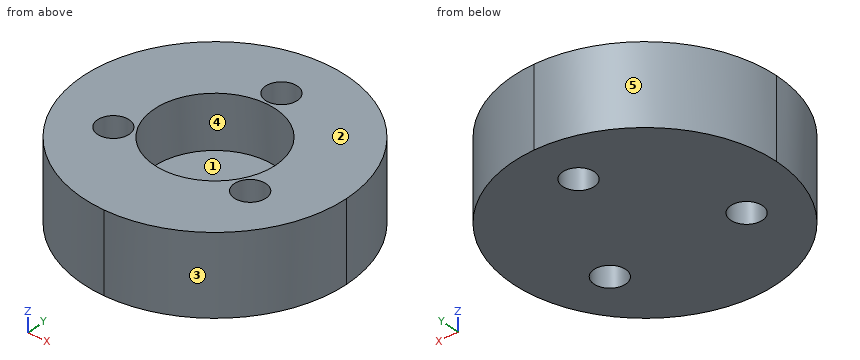
from build123d import *

# Parameters (mm, degrees)
SKETCH1_W                = 20
SKETCH1_H                = 20
SKETCH1_R                = 6
BOSS_EXTRUDE1_DEPTH      = 6
M2_CLEARANCE_HOLE1_D     = 2.4
M2_CLEARANCE_HOLE1_DEPTH = 10
M2_CLEARANCE_HOLE1_TIP   = 0.721032743
FILLET1_R                = 10
SKETCH4_R                = 4.6
CUT_EXTRUDE1_DEPTH       = 4


with BuildPart() as part:
    # Sketch1 → Boss-Extrude1 (new body)
    # profile 1 of 2: a face of its own
    with BuildSketch(Plane.XY):
        with Locations((10, 10)):
            Rectangle(SKETCH1_W, SKETCH1_H)
        with Locations((10, 10)):
            Circle(SKETCH1_R, mode=Mode.SUBTRACT)
    # profile 2 of 2: a face of its own
    with BuildSketch(Plane.XY):
        with Locations((10, 10)):
            Circle(SKETCH1_R)
    extrude(amount=BOSS_EXTRUDE1_DEPTH)

    # M2 Clearance Hole1
    with Locations(Plane.XY.offset(6)):
        with Locations((10, 16), (15.196152423, 7), (4.803847577, 7)):
            Hole(M2_CLEARANCE_HOLE1_D / 2, depth=M2_CLEARANCE_HOLE1_DEPTH)
            with Locations((0, 0, -(M2_CLEARANCE_HOLE1_DEPTH + M2_CLEARANCE_HOLE1_TIP / 2))):  # 118° drill point
                Cone(0, M2_CLEARANCE_HOLE1_D / 2, M2_CLEARANCE_HOLE1_TIP, mode=Mode.SUBTRACT)

    # Fillet1
    fillet1_edges = [part.edges().sort_by_distance(p)[0] for p in [
        (0, 0, 3),
        (20, 0, 3),
        (20, 20, 3),
        (0, 20, 3),
    ]]
    fillet(fillet1_edges, radius=FILLET1_R - 0.0001)  # a hair under: the kernel refuses the full size

    # Sketch4 → Cut-Extrude1 (cut)
    with BuildSketch(Plane.XY.offset(6)):
        with Locations((10, 10)):
            Circle(SKETCH4_R)
    extrude(amount=-CUT_EXTRUDE1_DEPTH, mode=Mode.SUBTRACT)


solid = part.part
Geometry check sheet. Reference: the model listing, model coordinates, mm. Face numbers are marked on the shaded views. A direction names the side the tool comes from. Round coordinates to 2 decimals unless told otherwise and drop trailing zeros. Order: outer loops, then holes, each group sorted by start corner. A loop starts at its lowest first (then second) coordinate and runs counter-clockwise, first axis right, second up. Notation, with made-up numbers: (-26, 13.25) - (1, 13.25) arc R7 cw to (1, 25.25) - close; hole circle Ø4 at (-12, 38). An arc over 180 degrees is marked (long way). One line per question, with ' | ' between items. Start each with the question number.
(1) Sectioned sample at C-C on x = 4.5. Record the cut outline in (y, z).
(2) Sectioned sample at B-B on y = 7. Record the cut outline in (x, z), and give its area (3 significant figures).
(3) Sectioned sample at A-A on z = 4.1. Count the separate pieces of the cut face and the enclosed holes in it, and give its area (3 significant figures).
(4) Release check for a two-part mould opening along X. For the marked faces 1, 2 and 3 record: released by +X, released by -X, zero draft, split by the parting line, or undercut.
(5) Access from +Z, -Z, +X, -X, +Y, -Y to the whole of each face (thin tool, end or side, straight path). Record for the marked faces 4 and 5.
(6) Sectioned sample at D-D on x = 11.5. Record the cut outline in (y, z), and give its area (3 significant figures).
(7) Thickness scan on L1, parallel to Y at x = 10, z = 4.4; L2, parallel to Y at x = 6.75, z = 4.55; L3, parallel to X at y = 13.5, z = 3.4. Record the ranges inside material, lowest first. Write a range as [from, to].
(8) Depth check by flat-ended pin: pin 1 Ø1 at (y, z) = (5.5, 5) entering from -X; pin 2 Ø4.5 at (x, y) = (9, 8) entering from +Z; pin 3 Ø1.4 at (x, y) = (4.8, 7) entering from +Z; pin 4 Ø2 at (x, z) = (2.5, 3.5) entering from +Y. Enter the tip coordinate at first touch or a pass-through.
Conclusion:
1) outline: (1.65, 0) - (5.84, 0) - (5.84, 6) - (1.65, 6) - close; (8.16, 0) - (18.35, 0) - (18.35, 6) - (8.16, 6) - close
2) outline: (0.46, 0) - (3.6, 0) - (3.6, 6) - (0.46, 6) - close; (6, 0) - (14, 0) - (14, 6) - (13.49, 6) - (13.49, 2) - (6.51, 2) - (6.51, 6) - (6, 6) - close; (16.4, 0) - (19.54, 0) - (19.54, 6) - (16.4, 6) - close | area: 57.8 mm2
3) separate pieces: 1 | enclosed holes: 4 | area: 234 mm2
4) face 1: undercut | face 2: zero draft | face 3: released by +X
5) face 4: +Z | face 5: +Z, -Z, -X, +Y
6) outline: (0.11, 0) - (19.89, 0) - (19.89, 6) - (14.35, 6) - (14.35, 2) - (5.65, 2) - (5.65, 6) - (0.11, 6) - close | area: 83.9 mm2
7) L1: y = [0, 5.4], [14.6, 14.8], [17.2, 20] | L2: y = [0.54, 6.74], [13.26, 19.46] | L3: x = [0.63, 7.02], [12.98, 19.37]
8) pin 1: stops at x = 0.83 | pin 2: stops at z = 2 | pin 3: passes through | pin 4: stops at y = 17.6
